Here's how the part is built. I have some questions about the finished solid (model axes, mm). A direction names the side the tool comes from. Give positions to 0.01 mm unless a question says otherwise; leave off trailing zeros. Loops run counter-clockwise (first coordinate to the right, second up) from the corner with the lowest first, then second, coordinate; pieces in that order, holes last.
Q1. Suppose I cut it at D-D (x = -8). List the corners of the cut face in (y, z) for me, and give its area (3 significant figures).
Q2. Suppose I cut it at C-C (z = 7). List the corners of the cut face in (x, y) for me.
Q3. Thinking about a two-plate mould opening in Y: for faces 5 (the face through (0, 29, 5)), 6 (the face through (-1.172, 8.923, 8.986)), 7 (the face through (6.8, 26.5, -4.1)), which applies, pulls with the +Y half, pulls with the -Y half, needs draft (parallel to the pull), parting line crosses it, or undercut?
Q4. Suppose I cut it at B-B (x = 0). List the corners of the cut face in (y, z) for me, and give its area (3 significant figures).
Q5. I need wall thicknesses on probe 1 along Z at (x, y) = (8, 25.15); probe 2 along Z at (x, y) = (-8, 26.8); probe 3 along Y at (x, z) = (0, 1.75). Which ranges of each line are inside material? Lowest first, please.
Q6. I'm going to push flat-ended pins straight in: P1, Ø1.5, axis at y = 27.5, z = 16.5, coming from the -X side; P2, Ø14, axis at x = -7, y = 5.5, coming from the +Z side; P3, Ø8, axis at x = 2.5, y = -7, coming from the -Z side; P4, Ø6, axis at y = 4, z = -1, coming from the +X side. Where does each tip first touch, or does it pass through?
Q7. For faces 1 (the face through (5, 24, 15)), 2 (the face through (0, 13, 0)), 3 (the face through (-4, 27, 15)), 4 (the face through (-2.38, -10.74, 3.94)), which set-ups out of +Z, -Z, +X, -X, +Y, -Y let a thin tool reach every point of the face, with its end or its side?
Q8. Suppose I cut it at A-A (y = 0). List the corners of the cut face in (x, z) for me.
```python
from build123d import *

# Parameters (mm, degrees)
CROQUIS1_W              = 45
CROQUIS1_H              = 28
CROQUIS1_R              = 11
SALIENTE_EXTRUIR1_DEPTH = 10
SALIENTE_EXTRUIR2_START = -2
CROQUIS2_R              = 11
CROQUIS2_R_2            = 9
SALIENTE_EXTRUIR2_DEPTH = 2
CROQUIS3_R              = 1.5
SALIENTE_EXTRUIR3_DEPTH = 5
CORTAR_EXTRUIR1_REACH   = 46.011
CORTAR_EXTRUIR2_REACH   = 53.196
CROQUIS5_W              = 10
CROQUIS5_H              = 10


with BuildPart() as part:
    # Croquis1 → Saliente-Extruir1 (new body)
    with BuildSketch(Plane(origin=(0, 0, 0), x_dir=(0, 1, 0), z_dir=(0, 0, 1))):
        with Locations((6.5, 0)):
            Rectangle(CROQUIS1_W, CROQUIS1_H)
        with Locations(Location((0, 0, 0), (0, 0, 270))):
            Circle(CROQUIS1_R, mode=Mode.SUBTRACT)
    extrude(amount=SALIENTE_EXTRUIR1_DEPTH)

    # Croquis2 → Saliente-Extruir2 (add)
    with BuildSketch(Plane.XY.offset(10).offset(SALIENTE_EXTRUIR2_START)):
        Circle(CROQUIS2_R)
        Circle(CROQUIS2_R_2, mode=Mode.SUBTRACT)
    extrude(amount=SALIENTE_EXTRUIR2_DEPTH)

    # Croquis3 → Saliente-Extruir3 (add)
    # profile 1 of 2: a face of its own
    with BuildSketch(Plane(origin=(0, 29, 0), x_dir=(1, 0, 0), z_dir=(0, 1, 0))):
        with BuildLine():
            Line((-9, -20), (9, -20))
            ThreePointArc((9, -20), (12.535533906, -18.535533906), (14, -15))
            Line((14, -15), (14, -10))
            Line((14, -10), (-14, -10))
            Line((-14, -10), (-14, -15))
            ThreePointArc((-14, -15), (-12.535533906, -18.535533906), (-9, -20))
        make_face()
        with Locations(Location((8, -15, 0), (0, 0, 180))):
            Circle(CROQUIS3_R, mode=Mode.SUBTRACT)
        with Locations((-8, -15)):
            Circle(CROQUIS3_R, mode=Mode.SUBTRACT)
    # profile 2 of 2: a face of its own
    with BuildSketch(Plane(origin=(0, 29, 0), x_dir=(1, 0, 0), z_dir=(0, 1, 0))):
        with BuildLine():
            Line((-14, 0), (14, 0))
            Line((14, 0), (14, 5))
            ThreePointArc((14, 5), (12.535533906, 8.535533906), (9, 10))
            Line((9, 10), (-9, 10))
            ThreePointArc((-9, 10), (-12.535533906, 8.535533906), (-14, 5))
            Line((-14, 5), (-14, 0))
        make_face()
        with Locations(Location((-8, 5, 0), (0, 0, 180))):
            Circle(CROQUIS3_R, mode=Mode.SUBTRACT)
        with Locations((8, 5)):
            Circle(CROQUIS3_R, mode=Mode.SUBTRACT)
    extrude(amount=-SALIENTE_EXTRUIR3_DEPTH)

    # Croquis4 → Cortar-Extruir1 (cut, up to next)
    with BuildSketch(Plane.XY.offset(20), mode=Mode.PRIVATE) as cortar_extruir1_sk1:
        Polygon((12, 29), (14, 27), (14, 29), align=None)
    cortar_extruir1_tool1 = extrude(cortar_extruir1_sk1.sketch, amount=-CORTAR_EXTRUIR1_REACH, mode=Mode.PRIVATE) & part.part
    # Croquis4 → Cortar-Extruir1 (cut, up to next)
    with BuildSketch(Plane.XY.offset(20), mode=Mode.PRIVATE) as cortar_extruir1_sk2:
        Polygon((-14, 27), (-14, 29), (-12, 29), align=None)
    cortar_extruir1_tool2 = extrude(cortar_extruir1_sk2.sketch, amount=-CORTAR_EXTRUIR1_REACH, mode=Mode.PRIVATE) & part.part
    add(cortar_extruir1_tool1.solids().sort_by_distance((13.333333, 28.333333, 20))[0], mode=Mode.SUBTRACT)
    add(cortar_extruir1_tool2.solids().sort_by_distance((-13.333333, 28.333333, 20))[0], mode=Mode.SUBTRACT)

    # Croquis5 → Cortar-Extruir2 (cut, up to next)
    with BuildSketch(Plane(origin=(0, 29, 0), x_dir=(1, 0, 0), z_dir=(0, 1, 0)), mode=Mode.PRIVATE) as cortar_extruir2_sk1:
        with Locations((-9, -15)):
            Rectangle(CROQUIS5_W, CROQUIS5_H)
    cortar_extruir2_tool1 = extrude(cortar_extruir2_sk1.sketch, amount=-CORTAR_EXTRUIR2_REACH, mode=Mode.PRIVATE) & part.part
    add(cortar_extruir2_tool1.solids().sort_by_distance((-9, 29, 15))[0], mode=Mode.SUBTRACT)


solid = part.part
```
Solutions:
1. outline: (-16, 0) - (-7.55, 0) - (-7.55, 8) - (-4.12, 8) - (-4.12, 10) - (-16, 10) - close; (4.12, 8) - (7.55, 8) - (7.55, 0) - (24, 0) - (24, -3.5) - (29, -3.5) - (29, 10) - (4.12, 10) - close; (24, -10) - (29, -10) - (29, -6.5) - (24, -6.5) - close
1. area: 348 mm2
2. outline: (-14, -16) - (14, -16) - (14, 27) - (12, 29) - (-12, 29) - (-14, 27) - close; hole circle Ø22 at (0, 0)
3. face 5: pulls with the +Y half
3. face 6: undercut
3. face 7: needs draft
4. outline: (-16, 0) - (-11, 0) - (-11, 8) - (-9, 8) - (-9, 10) - (-16, 10) - close; (9, 8) - (11, 8) - (11, 0) - (24, 0) - (24, -10) - (29, -10) - (29, 20) - (24, 20) - (24, 10) - (9, 10) - close
4. area: 338 mm2
5. probe 1: z = -10 to -6.5, -3.5 to 13.5, 16.5 to 20
5. probe 2: z = -10 to -6.5, -3.5 to 10
5. probe 3: y = -16 to -11, 11 to 29
6. P1: stops at x = -4
6. P2: stops at z = 10
6. P3: stops at z = 0
6. P4: stops at x = 14
7. face 1: +Z, +X, -X, -Y
7. face 2: -Z, +X, -X, -Y
7. face 3: +Z, -X, +Y, -Y
7. face 4: -Z
8. outline: (-14, 0) - (-11, 0) - (-11, 8) - (-9, 8) - (-9, 10) - (-14, 10) - close; (9, 8) - (11, 8) - (11, 0) - (14, 0) - (14, 10) - (9, 10) - close
